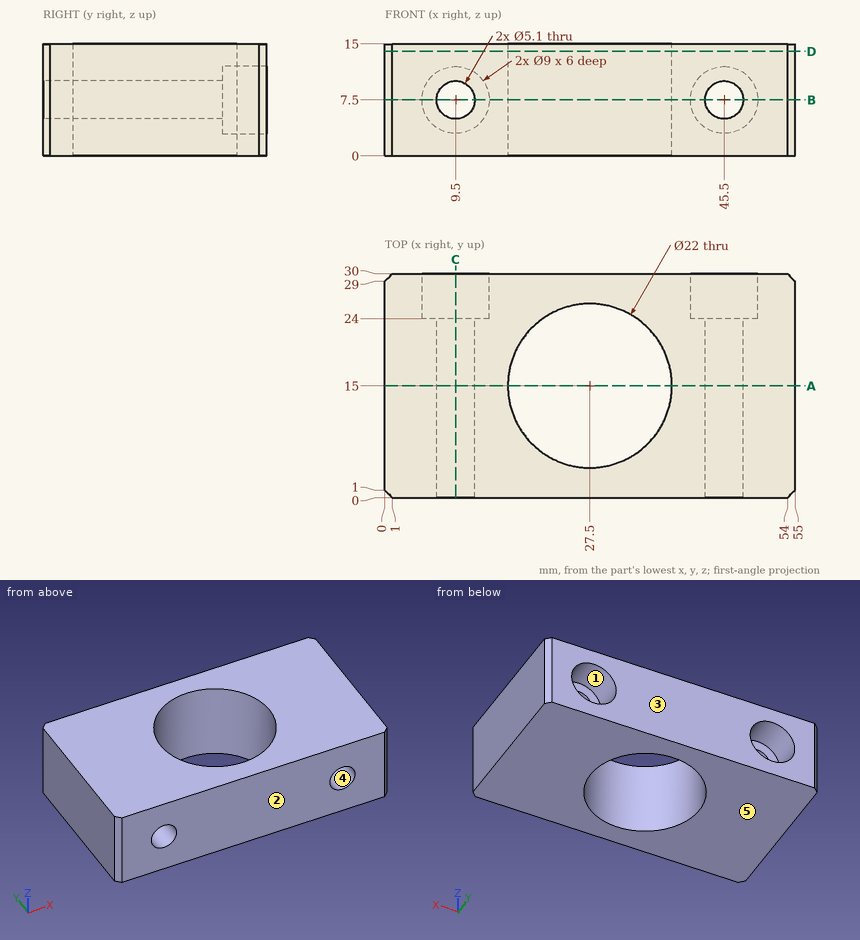
Geometry check sheet. Reference: drawing and pictorial views, mm from the part's lowest x, y, z. A direction names the side the tool comes from. Coordinates: 2 decimals unless noted, no trailing zeros. Order: outer loops, then holes, each group sorted by start corner. A loop starts at its lowest first (then second) coordinate and runs counter-clockwise, first axis right, second up.
Item 1: Depth check by flat-ended pin: pin 1 (13 mm diameter, centred on x = 27.5, y = 15, fed in from +Z). Enter the tip coordinate at first touch or a pass-through.
Item 2: Section check C-C (x = 9.5). Enter the section's corners in (y, z), plus the area to 3 significant figures.
Item 3: Section check B-B (z = 7.5). Enter the section's corners in (x, y).
Item 4: Section check D-D (z = 14). Enter the section's corners in (x, y), plus the area to 3 significant figures.
Item 5: Scan lines: line 1 along X through (y, z) = (28.6, 7.5); line 2 along Z through (x, y) = (45.5, 10); line 3 along X through (y, z) = (3.75, 7). Record each from-to range of solid material in increasing order.
Item 6: Tool access check on the marked faces 1 and 2. Record the directions out of +Z, -Z, +X, -X, +Y, -Y that give a thin tool (end or side, any length) a straight path to the whole face; none if there is none.
Item 7: Section check A-A (y = 15). Enter the section's corners in (x, z), plus the area to 3 significant figures.
Item 8: Mould release check, pull along Z, two halves, no side actions. Record for the marked faces 3, 4 and 5: released by +Z, released by -Z, zero draft, split by the parting line, or undercut.
Check sheet entries:
1. pin 1: passes through
2. outline: (0, 0) - (30, 0) - (30, 3) - (24, 3) - (24, 4.95) - (0, 4.95) - close; (0, 10.05) - (24, 10.05) - (24, 12) - (30, 12) - (30, 15) - (0, 15) - close
2. area: 274 mm2
3. outline: (0, 1) - (1, 0) - (6.95, 0) - (6.95, 24) - (5, 24) - (5, 30) - (1, 30) - (0, 29) - close; (12.05, 0) - (42.95, 0) - (42.95, 24) - (41, 24) - (41, 30) - (14, 30) - (14, 24) - (12.05, 24) - close; (48.05, 0) - (54, 0) - (55, 1) - (55, 29) - (54, 30) - (50, 30) - (50, 24) - (48.05, 24) - close; hole circle Ø22 at (27.5, 15)
4. outline: (0, 1) - (1, 0) - (54, 0) - (55, 1) - (55, 29) - (54, 30) - (1, 30) - (0, 29) - close; hole circle Ø22 at (27.5, 15)
4. area: 1,270 mm2
5. line 1: x = 0 to 5, 14 to 41, 50 to 55
5. line 2: z = 0 to 4.95, 10.05 to 15
5. line 3: x = 0 to 7, 12 to 43, 48 to 55
6. face 1: +Y
6. face 2: +Z, -Z, +X, -X, -Y
7. outline: (0, 0) - (16.5, 0) - (16.5, 15) - (0, 15) - close; (38.5, 0) - (55, 0) - (55, 15) - (38.5, 15) - close; hole circle Ø5.1 at (9.5, 7.5); hole circle Ø5.1 at (45.5, 7.5)
7. area: 454 mm2
8. face 3: zero draft
8. face 4: undercut
8. face 5: released by -Z
